```python
from build123d import *

# Parameters (mm, degrees)
F0_R      = 2
F1_DEPTH  = 2
F2_W      = 24
F2_H      = 8
F3_DEPTH  = 10
F5_DEPTH  = 8
F7_DEPTH  = 40
F9_DEPTH  = 25
F11_DEPTH = 24
F13_DEPTH = 4
F14_R     = 2
F15_DEPTH = 4
F17_DEPTH = 4


with BuildPart() as f1:
    # F0 (on Top) → F1 (new body)
    with BuildSketch(Plane.XY):
        with BuildLine():
            Line((40, 20), (4, 20))
            ThreePointArc((4, 20), (1.1715728753, 18.8284271247), (0, 16))
            Line((0, 16), (0, -8))
            ThreePointArc((0, -8), (4, -12), (8, -8))
            Line((8, -8), (8, 0))
            Line((8, 0), (40, 0))
            ThreePointArc((40, 0), (42.8284271247, 1.1715728753), (44, 4))
            Line((44, 4), (44, 16))
            ThreePointArc((44, 16), (42.8284271247, 18.8284271247), (40, 20))
        make_face()
        with Locations((4, -8)):
            Circle(F0_R, mode=Mode.SUBTRACT)
        with Locations((4, 16)):
            Circle(F0_R, mode=Mode.SUBTRACT)
        with Locations((40, 4)):
            Circle(F0_R, mode=Mode.SUBTRACT)
        with Locations((40, 16)):
            Circle(F0_R, mode=Mode.SUBTRACT)
    extrude(amount=F1_DEPTH)

    # F2 (on face) → F3 (join)
    with BuildSketch(Plane.XY.offset(2)):
        with Locations((20, 4)):
            Rectangle(F2_W, F2_H)
    extrude(amount=F3_DEPTH)

    # F4 (on face) → F5 (join)
    with BuildSketch(Plane.XZ):
        with BuildLine():
            Line((32, 2), (35, 2))
            ThreePointArc((35, 2), (32.8786796564, 2.8786796564), (32, 5))
            Line((32, 5), (32, 2))
        make_face()
        with BuildLine():
            Line((5, 2), (8, 2))
            Line((8, 2), (8, 5))
            ThreePointArc((8, 5), (7.1213203436, 2.8786796564), (5, 2))
        make_face()
    extrude(amount=-F5_DEPTH)

    # F6 (on face) → F7 (join)
    with BuildSketch(Plane.YZ.offset(44)):
        with BuildLine():
            ThreePointArc((11, 2), (8.8786796564, 2.8786796564), (8, 5))
            Line((8, 5), (8, 2))
            Line((8, 2), (11, 2))
        make_face()
    extrude(amount=-F7_DEPTH)

    # F8 (on face) → F9 (cut)
    with BuildSketch(Plane.XZ):
        with BuildLine():
            ThreePointArc((5, 2), (7.1213203436, 2.8786796564), (8, 5))
            Line((8, 5), (3.8540177047, 5))
            Line((3.8540177047, 5), (3.8540177047, 2))
            Line((3.8540177047, 2), (5, 2))
        make_face()
        with BuildLine():
            Line((44, 5), (32, 5))
            ThreePointArc((32, 5), (32.8786796564, 2.8786796564), (35, 2))
            Line((35, 2), (40, 2))
            Line((40, 2), (44, 2))
            Line((44, 2), (44, 5))
        make_face()
    extrude(amount=-F9_DEPTH, mode=Mode.SUBTRACT)

    # F10 (on face) → F11 (join)
    with BuildSketch(Plane.YZ.offset(32)):
        Polygon((22.5059458821, 36.1346721534), (0, 12), (8, 12), (8, 14.7138329376), (24.2451953819, 32.1346721534), (38.5059458821, 32.1346721534), (38.5059458821, 36.1346721534), align=None)
    extrude(amount=-F11_DEPTH)

    # F12 (on face) → F13 (cut)
    with BuildSketch(Plane(origin=(0, -5.9853843016, 5.5814611575), x_dir=(1, 0, 0), z_dir=(0, -0.7313537016, 0.6819983601))):
        with BuildLine():
            Line((26, 18.7762444194), (26, 32.7762444194))
            ThreePointArc((26, 32.7762444194), (24, 34.7762444194), (22, 32.7762444194))
            Line((22, 32.7762444194), (22, 18.7762444194))
            ThreePointArc((22, 18.7762444194), (24, 16.7762444194), (26, 18.7762444194))
        make_face()
    extrude(amount=-F13_DEPTH, mode=Mode.SUBTRACT)

    # F14 (on face) → F15 (join)
    with BuildSketch(Plane(origin=(0, -5.9853843016, 5.5814611575), x_dir=(1, 0, 0), z_dir=(0, -0.7313537016, 0.6819983601))):
        with BuildLine():
            Line((8, 30.7762444194), (4, 30.7762444194))
            ThreePointArc((4, 30.7762444194), (-2, 24.7762444194), (4, 18.7762444194))
            Line((4, 18.7762444194), (8, 18.7762444194))
            Line((8, 18.7762444194), (8, 30.7762444194))
        make_face()
        with Locations((4, 24.7762444194)):
            Circle(F14_R, mode=Mode.SUBTRACT)
    extrude(amount=-F15_DEPTH)

    # F16 (on face) → F17 (cut)
    with BuildSketch(Plane.XY.offset(36.1346721534)):
        with BuildLine():
            ThreePointArc((14, 38.5059458821), (20, 32.5059458821), (26, 38.5059458821))
            Line((26, 38.5059458821), (14, 38.5059458821))
        make_face()
    extrude(amount=-F17_DEPTH, mode=Mode.SUBTRACT)


solid = f1.part
```
Source: CAD feature listing. Evaluate the final solid. Frame: model axes, mm. A direction names the side the tool comes from. Give positions to 0.01 mm unless a question says otherwise; leave off trailing zeros. Write each loop counter-clockwise with the first axis right and the second up, starting at its lowest first coordinate (ties: lowest second). Pieces come first, ordered by that corner, then holes.
1. Section query B-B (x = 25). Return the cut outline in (y, z), then the cut area to 3 significant figures.
2. Material intervals for line 1 along Y through (x, z) = (40, 1.1); line 2 along X through (y, z) = (12.5, 20); line 3 along X through (y, z) = (27.5, 34), sorted ascending.
3. Pull-direction query (Z, two-part tool) for faces 1 (the face through (20, 30, 32.135)), 2 (the face through (19.868, 32.507, 34.163)), 3 (the face through (-2, 12.4, 22.5)), 4 (the face through (20, 8, 10)); classes: +Z half, -Z half, draft (parallel to the pull), parting line (faces both ways), or undercut.
4. Section query C-C (x = 20). Return the cut outline in (y, z).
5. Access query for faces 5 (the face through (6.03, 16.45, 26.74)), 6 (the face through (4, 18, 1)), 7 (the face through (26, 13, 23)), 8 (the face through (0, 4, 1)). Directions: +Z, -Z, +X, -X, +Y, -Y. A direction counts if a zero-diameter tool reaches every point of the face in a straight line with its end or side. Return the directions, or none.
6. Section query D-D (z = 9). Return the cut outline in (x, y), then the cut area to 3 significant figures.
7. First-contact query: pin 1 (3.5 mm diameter, centred on x = 22.5, z = 8.5, fed in from -Y); pin 2 (1 mm diameter, centred on y = -1, z = 1, fed in from -X); pin 3 (16 mm diameter, centred on x = 25, y = 1.5, fed in from +Z); pin 4 (1.5 mm diameter, centred on y = -1.5, z = 12, fed in from +X). Flat tips, straight axial feed; report the tip coordinate or a pass-through.
8. Section query A-A (y = -9). Return the cut outline in (x, z), then the cut area to 3 significant figures.
Output values:
1. outline: (0, 0) - (20, 0) - (20, 2) - (11, 2) arc R3 cw to (8, 5) - (8, 14.71) - (8.56, 15.32) - (5.64, 18.05) - (0, 12) - close; (17.55, 30.82) - (20.47, 28.09) - (24.25, 32.13) - (35.19, 32.13) - (35.19, 36.13) - (22.51, 36.13) - close
1. area: 224 mm2
2. line 1: y = 0 to 2, 6 to 14, 18 to 20
2. line 2: x = -1.78 to 2.83, 5.17 to 22, 26 to 32
2. line 3: x = 8 to 32
3. face 1: -Z half
3. face 2: draft
3. face 3: undercut
3. face 4: undercut
4. outline: (0, 0) - (20, 0) - (20, 2) - (11, 2) arc R3 cw to (8, 5) - (8, 14.71) - (24.25, 32.13) - (32.51, 32.13) - (32.51, 36.13) - (22.51, 36.13) - (0, 12) - close
5. face 5: +Z, -X, +Y
5. face 6: -Z
5. face 7: none
5. face 8: -Z, -X, +Y, -Y
6. outline: (8, 0) - (32, 0) - (32, 8) - (8, 8) - close
6. area: 192 mm2
7. pin 1: stops at y = 0
7. pin 2: stops at x = 0
7. pin 3: stops at z = 22.12
7. pin 4: passes through
8. outline: (0.13, 0) - (2.27, 0) - (2.27, 2) - (0.13, 2) - close; (5.73, 0) - (7.87, 0) - (7.87, 2) - (5.73, 2) - close
8. area: 8.56 mm2
